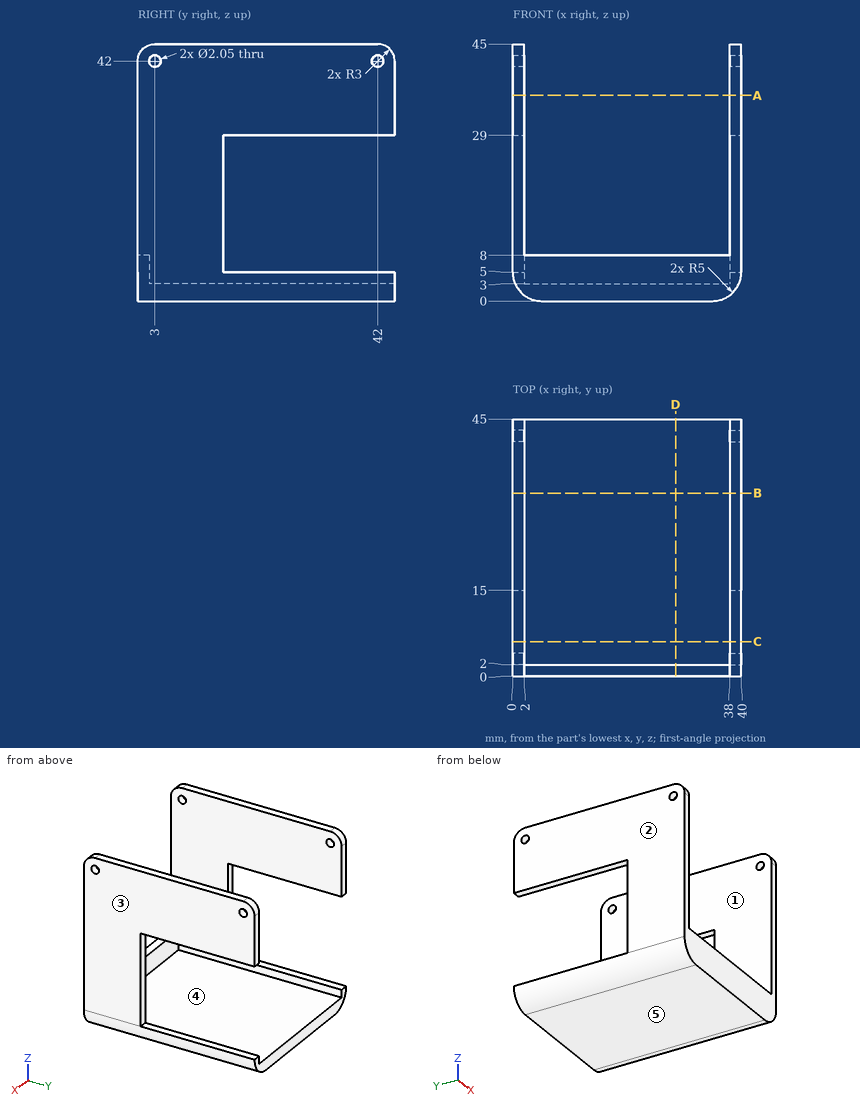
Drawing for the job (mm, zero at the part's lowest x, y, z). A direction names the side the tool comes from. Round coordinates to 2 decimals unless told otherwise and drop trailing zeros. Loops run counter-clockwise (first coordinate to the right, second up) from the corner with the lowest first, then second, coordinate; pieces in that order, holes last. Notation, with made-up numbers: M -13,27 L 41,27 A25 cw 41,45 Z; hole C -17.5,4 d2. An arc over 180 degrees is marked long. Use a Markdown table: item, result. Add a question column.
(1) Cut at A-A (z = 36). Give the cut face in (x, y), and give its area (3 significant figures).
(2) Cut at C-C (y = 6). Give the cut face in (x, z), and give its area (3 significant figures).
(3) Pull direction X, two halves, no side cores. Call the marked faces 1, 2 and 3: +X half, -X half, draft (parallel to the pull), parting line (faces both ways), or undercut.
(4) Drill centre lines: line 1 (Y direction, x = 1.5, z = 42) (3 decimals); line 2 (X direction, y = 28, z = 37); line 3 (Z direction, x = 31.5, y = 31.5). Where is each one in solid material? Low to high.
(5) Cut at D-D (x = 28.5). Give the cut face in (y, z).
(6) Flat gauge pins, fed straight in: pin 1 (1.5 mm diameter, centred on x = 25, z = 6, fed in from +Y); pin 2 (5 mm diameter, centred on x = 6.5, y = 24.5, fed in from +Z); pin 3 (1.6 mm diameter, centred on x = 1.5, z = 18, fed in from +Y). Where does each tip first touch, or does it go through?
(7) Cut at B-B (y = 32). Give the cut face in (x, z), and give its area (3 significant figures).
(8) Which spindle directions (+Z, -Z, +X, -X, +Y, -Y) get a long thin tool onto all of the face, cutting with end or side? Do the marked faces 4 and 5. Say none if no direction does.
Geometry says:
| question | item | result |
|---|---|---|
| 1 | outline | M 0,0 L 2,0 L 2,45 L 0,45 Z; M 38,0 L 40,0 L 40,45 L 38,45 Z |
| 1 | area | 180 mm² |
| 2 | outline | M 0,5 A5 ccw 5,0 L 35,0 A5 ccw 40,5 L 40,45 L 38,45 L 38,3 L 2,3 L 2,45 L 0,45 Z |
| 2 | area | 277 mm² |
| 3 | face 1 | undercut |
| 3 | face 2 | -X half |
| 3 | face 3 | +X half |
| 4 | line 1 | y = 0 to 1.975, 4.025 to 40.975, 43.025 to 45 |
| 4 | line 2 | x = 0 to 2, 38 to 40 |
| 4 | line 3 | z = 0 to 3 |
| 5 | outline | M 0,0 L 45,0 L 45,3 L 2,3 L 2,8 L 0,8 Z |
| 6 | pin 1 | stops at y = 2 |
| 6 | pin 2 | stops at z = 3 |
| 6 | pin 3 | stops at y = 15 |
| 7 | outline | M 0,5 A5 ccw 5,0 L 35,0 A5 ccw 40,5 L 38,5 L 38,3 L 2,3 L 2,5 Z; M 0,29 L 2,29 L 2,45 L 0,45 Z; M 38,29 L 40,29 L 40,45 L 38,45 Z |
| 7 | area | 181 mm² |
| 8 | face 4 | +Z, +Y |
| 8 | face 5 | -Z, +X, -X, +Y, -Y |
